For this review, use the dimensioned drawing (mm, ordinates from the lowest corner) and the shaded views. A direction names the side the tool comes from. Give positions to 0.01 mm unless a question says otherwise; leave off trailing zeros. Write each loop counter-clockwise with the first axis right and the second up, starting at its lowest first coordinate (ties: lowest second). Pieces come first, ordered by that corner, then holes. Notation, with made-up numbers: (-9, -36.5) - (10, -36.5) arc R24 cw to (10, -16.5) - close; hole circle Ø4 at (61.25, -25). An arc over 180 degrees is marked (long way). Use a Markdown table: item, result. Add a question column.
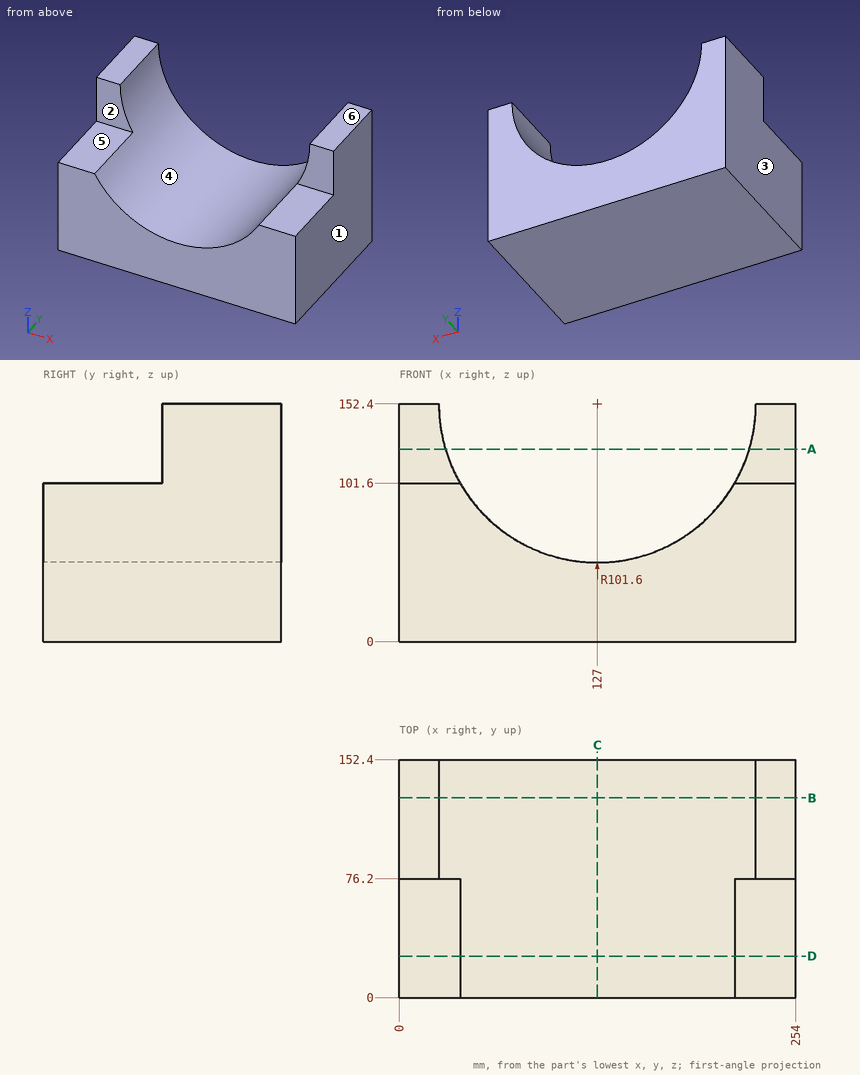
(1) Add section C-C (x = 127). State the section outline as (y, z) points, and give its area (3 significant figures).
(2) Insertion check: pin 1 (19.5 mm diameter, centred on x = 230, y = 39, fed in from +Z). The pin has a flat end and moves straight along its axis. Give the tip position at first contact, or say it passes through.
(3) Tool access review of the marked faces 5 and 6: name each direction out of +Z, -Z, +X, -X, +Y, -Y from which nothing blocks a thin tool from reaching the whole face with its end or side.
(4) Add section D-D (y = 26.5). State the section outline as (x, z) points, and give its area (3 significant figures).
(5) Mouldability with a two-part tool opening along X and no side actions: class the marked faces 1, 2, 3 and 4 as +X half, -X half, draft (parallel to the pull), parting line (faces both ways), or undercut.
(6) Add section B-B (y = 128). State the section outline as (x, z) points, and give its area (3 significant figures).
(7) Add section A-A (z = 123.5). State the section outline as (x, y) points, and give its area (3 significant figures).
(8) For line 1 along Z through (x, y) = (226.5, 44); line 2 along X through (y, z) = (22.5, 64.5); line 3 along Y through (x, z) = (233, 124), list the stretches that pass through material, from the lowest coordinate up.
Answers follow:
| question | item | result |
|---|---|---|
| 1 | outline | (0, 0) - (152.4, 0) - (152.4, 50.8) - (0, 50.8) - close |
| 1 | area | 7,740 mm^2 |
| 2 | pin 1 | z = 101.6 |
| 3 | face 5 | +Z, +X, -X, -Y |
| 3 | face 6 | +Z, +X, -X, +Y, -Y |
| 4 | outline | (0, 0) - (254, 0) - (254, 101.6) - (214.99, 101.6) arc R101.6 cw to (39.01, 101.6) - (0, 101.6) - close |
| 4 | area | 19,500 mm^2 |
| 5 | face 1 | +X half |
| 5 | face 2 | draft |
| 5 | face 3 | -X half |
| 5 | face 4 | undercut |
| 6 | outline | (0, 0) - (254, 0) - (254, 152.4) - (228.6, 152.4) arc R101.6 cw to (25.4, 152.4) - (0, 152.4) - close |
| 6 | area | 22,500 mm^2 |
| 7 | outline | (0, 76.2) - (29.6, 76.2) - (29.6, 152.4) - (0, 152.4) - close; (224.4, 76.2) - (254, 76.2) - (254, 152.4) - (224.4, 152.4) - close |
| 7 | area | 4,510 mm^2 |
| 8 | line 1 | 0 to 101.6 |
| 8 | line 2 | 0 to 76.05, 177.95 to 254 |
| 8 | line 3 | 76.2 to 152.4 |
